Here's the drawing with two shaded views (mm, measured from the low corner). I have some questions. A direction names the side the tool comes from. Round coordinates to 2 decimals unless told otherwise and drop trailing zeros. Order: outer loops, then holes, each group sorted by start corner. A loop starts at its lowest first (then second) coordinate and runs counter-clockwise, first axis right, second up.
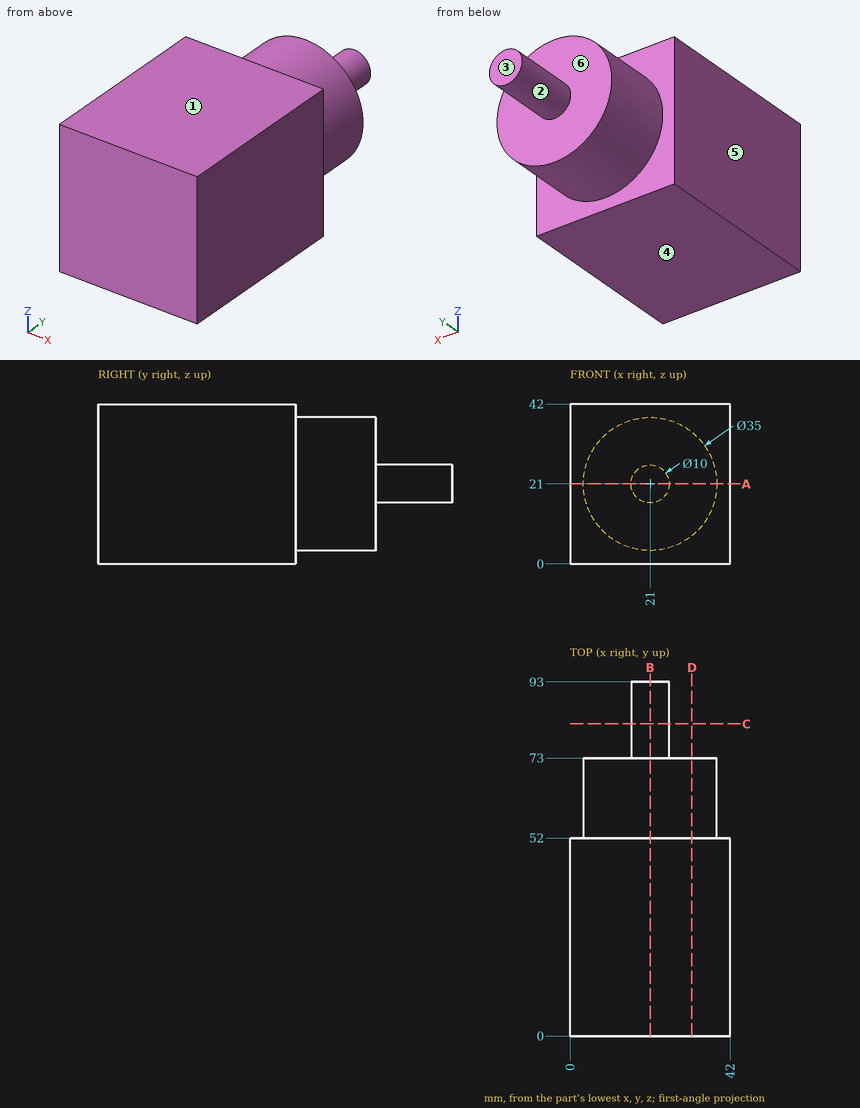
Q1. Imagine slicing it at D-D, the plane x = 32. Please give me the cut outline in (y, z), then the cut area to 3 significant figures.
Q2. Imagine slicing it at B-B, the plane x = 21. Please give me the cut outline in (y, z), then the cut area to 3 significant figures.
Q3. I need wall thicknesses on L1, parallel to Y at x = 3, z = 26.5; L2, parallel to Z at x = 21, y = 82; L3, parallel to Y at x = 20, z = 12.5. Which ranges of each line are inside material? Lowest first, please.
Q4. For the marked faces 5 and 6, which set-ups out of +Z, -Z, +X, -X, +Y, -Y let a thin tool reach every point of the face, with its end or its side?
Q5. Imagine slicing it at A-A, the plane z = 21. Please give me the cut outline in (x, y), then the cut area to 3 significant figures.
Q6. We'd pull the mould along Z, two halves only. Please class the marked faces 1, 2, 3 and 4: released by +Z, released by -Z, zero draft, split by the parting line, or undercut.
Q7. Imagine slicing it at C-C, the plane y = 82. Please give me the cut outline in (x, z).
Q8. For P1, Ø6, axis at y = 74, z = 37.5, coming from the +X side; P2, Ø12, axis at y = 70.5, z = 16.5, coming from the +X side, each with a flat end and sliding along its axis, tell me the tip position at first contact or that it passes through.
Filled in:
1. outline: (0, 0) - (52, 0) - (52, 7.39) - (73, 7.39) - (73, 34.61) - (52, 34.61) - (52, 42) - (0, 42) - close
1. area: 2,760 mm2
2. outline: (0, 0) - (52, 0) - (52, 3.5) - (73, 3.5) - (73, 16) - (93, 16) - (93, 26) - (73, 26) - (73, 38.5) - (52, 38.5) - (52, 42) - (0, 42) - close
2. area: 3,120 mm2
3. L1: y = 0 to 52
3. L2: z = 16 to 26
3. L3: y = 0 to 73
4. face 5: +Z, -Z, -X, +Y, -Y
4. face 6: +Y
5. outline: (0, 0) - (42, 0) - (42, 52) - (38.5, 52) - (38.5, 73) - (26, 73) - (26, 93) - (16, 93) - (16, 73) - (3.5, 73) - (3.5, 52) - (0, 52) - close
5. area: 3,120 mm2
6. face 1: released by +Z
6. face 2: split by the parting line
6. face 3: zero draft
6. face 4: released by -Z
7. outline: circle Ø10 at (21, 21)
8. P1: stops at x = 31.92
8. P2: stops at x = 38.5
